The model under review builds one solid part; all positions refer to its coordinate system, in mm. A direction names the side the tool comes from. Give positions to 0.01 mm unless a question says otherwise; leave off trailing zeros. Loops run counter-clockwise (first coordinate to the right, second up) from the corner with the lowest first, then second, coordinate; pieces in that order, holes last. Notation, with made-up numbers: M 87.5,58.5 L 127.5,58.5 A24 ccw 127.5,79.5 Z; hole C 56.5,1.5 d1. An arc over 180 degrees is marked long. Return JSON: item names as keys, results as strings. Group by question number.
```python
from build123d import *

# Parameters (mm, degrees)
F2_R     = 4.7625
F3_DEPTH = 9.525
F4_R     = 0.9525
F5_DEPTH = 22.225


with BuildPart() as f1:
    # F0 (on Front) → F1 (revolve)
    with BuildSketch(Plane.XZ):
        with BuildLine():
            Line((0, 58.42), (0, 0))
            Line((0, 0), (1.905, 0))
            Line((1.905, 0), (27.03371, 41.168312))
            ThreePointArc((27.03371, 41.168312), (27.127747, 46.301084), (22.697647, 48.895))
            Line((22.697647, 48.895), (8.504043, 48.895))
            Line((8.504043, 48.895), (8.504043, 58.42))
            Line((8.504043, 58.42), (0, 58.42))
        make_face()
    revolve(axis=Axis((0, 0, 29.21), (0, 0, -1)))

    # F2 (on face) → F3 (cut)
    with BuildSketch(Plane.XY.offset(58.42)):
        Circle(F2_R)
    extrude(amount=-F3_DEPTH, mode=Mode.SUBTRACT)

    # F4 (on face) → F5 (cut)
    with BuildSketch(Plane(origin=(0, 0, 0), x_dir=(1, 0, 0), z_dir=(0, 0, -1))):
        Circle(F4_R)
    extrude(amount=-F5_DEPTH, mode=Mode.SUBTRACT)


solid = f1.part
```
(1) Add section C-C (z = 51.5). Write out the cut boundary in (x, y) (1 decimal), and give its area (3 significant figures).
(2) For probe 1 along Y at (x, z) = (0, 55.75); probe 2 along Y at (x, z) = (0, 8.5); probe 3 along X at (y, z) = (0, 10.5), list the stretches that pass through material, from the lowest coordinate up.
(3) For pin 1 (3 mm diameter, centred on x = 7.5, z = 36.5, fed in from -Y); pin 2 (2 mm diameter, centred on x = -0.5, y = 0.5, fed in from -Z); pin 3 (1.5 mm diameter, centred on x = 0, y = 0, fed in from -Z) (3 decimals); pin 4 (8 mm diameter, centred on x = -9.5, z = 15.5, fed in from -Y), all flat-tipped, find the tip position at first contact; note any pin that passes through.
(4) Add section D-D (z = 32.5). Write out the cut boundary in (x, y).
(5) For faces 1 (the cylindrical face through (-8.496, -0.374, 53.724)), 2 (the cylindrical face through (-0.21, 0.93, 10.96)), 3 (the flat face through (-1, 1, 0)), list the 3-axis set-ups (+Z, -Z, +X, -X, +Y, -Y) from which the entire face can be reached by the end or side of a thin tool; tool diameter is ignored.
(6) Add section A-A (y = 0). Write out the cut boundary in (x, z) (1 decimal).
(7) Mouldability with a two-part tool opening along Y and no side actions: class faces 4 (the cylindrical face through (-3.78, -2.9, 53.72)), 5 (the conical face through (-2.57, 11.571, 16.298)), 6 (the flat face through (4, 4, 58.42)) as released by +Y, released by -Y, zero draft, split by the parting line, or undercut.
Verdict:
{
 "1": {"outline": "C 0,0 d17; hole C 0,0 d9.5", "area": "156 mm²"},
 "2": {"probe 1": "y = -8.5 to -4.76, 4.76 to 8.5", "probe 2": "y = -7.09 to -0.95, 0.95 to 7.09", "probe 3": "x = -8.31 to -0.95, 0.95 to 8.31"},
 "3": {"pin 1": "stops at y = -24.05", "pin 2": "stops at z = 0", "pin 3": "stops at z = 22.225", "pin 4": "stops at y = -11.28"},
 "4": {"outline": "C 0,0 d43.49"},
 "5": {"face 1": "+Z", "face 2": "-Z", "face 3": "-Z, +X, -X, +Y, -Y"},
 "6": {"outline": "M -27,41.2 L -1.9,0 L -1,0 L -1,22.2 L 1,22.2 L 1,0 L 1.9,0 L 27,41.2 A5.1 ccw 22.7,48.9 L 8.5,48.9 L 8.5,58.4 L 4.8,58.4 L 4.8,48.9 L -4.8,48.9 L -4.8,58.4 L -8.5,58.4 L -8.5,48.9 L -22.7,48.9 A5.1 ccw Z"},
 "7": {"face 4": "undercut", "face 5": "split by the parting line", "face 6": "zero draft"}
}
